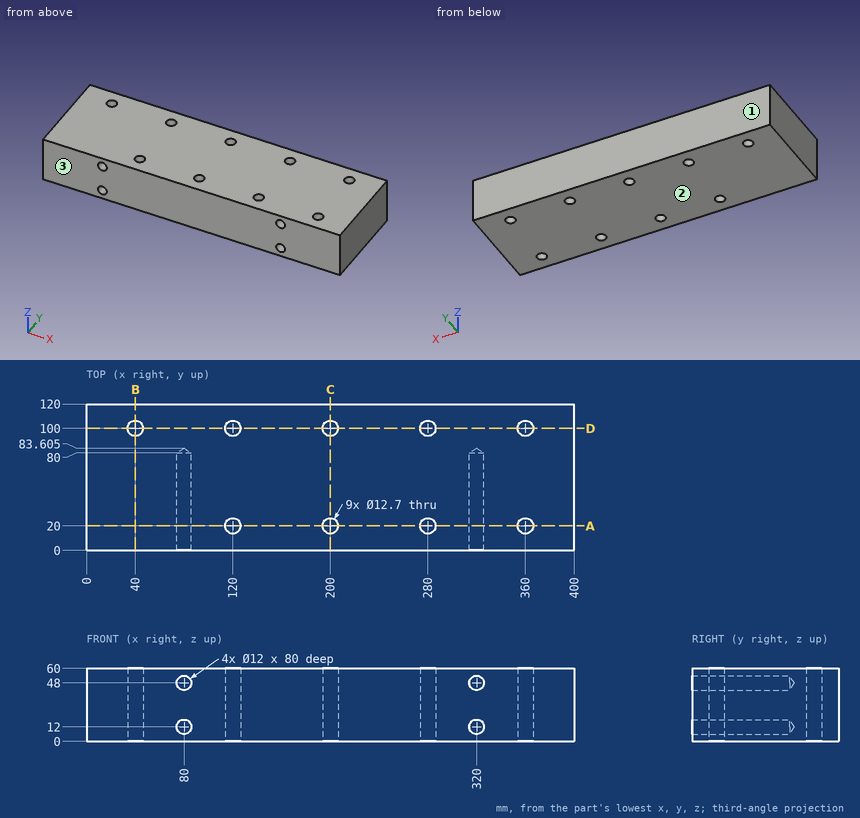
The drawing under review shows one solid part. Ordinate dimensions are in mm from its lowest x, y, z. Coordinates: 2 decimals unless noted, no trailing zeros. Order: outer loops, then holes, each group sorted by start corner. A loop starts at its lowest first (then second) coordinate and runs counter-clockwise, first axis right, second up. Notation, with made-up numbers: (8, 78) -> (48, 78) arc R20 cw to (48, 100) -> close; hole circle Ø8 at (-36, -31.75). An arc over 180 degrees is marked (long way). Answer in a Markdown table with one row per item. Add a question column.
Item 1: To check wall thickness, follow probe 1 along X at (y, z) = (56, 12); probe 2 along Z at (x, y) = (80, 62); probe 3 along Y at (x, z) = (360, 31). State the ranges of each line that lie inside material, in increasing order.
Item 2: Mouldability with a two-part tool opening along Y and no side actions: class the marked faces 1, 2 and 3 as +Y half, -Y half, draft (parallel to the pull), parting line (faces both ways), or undercut.
Item 3: We need section B-B on x = 40. Write out the cut boundary in (y, z).
Item 4: We need section D-D on y = 100. Write out the cut boundary in (x, z).
Item 5: We need section C-C on x = 200. Write out the cut boundary in (y, z), plus the area to 3 significant figures.
Item 6: We need section A-A on y = 20. Give the number of separate pieces and of enclosed holes in the cut face, plus the area to 3 significant figures.
Item 7: Clearance check with flat-ended pins moving along their axes: pin 1 (16.5 mm diameter, centred on x = 120, y = 20, fed in from -Z); pin 2 (7.5 mm diameter, centred on x = 200, y = 20, fed in from +Z); pin 3 (11 mm diameter, centred on x = 320, z = 48, fed in from -Y). State where each tip first meets the part, or that it passes through.
Final values:
| question | item | result |
|---|---|---|
| 1 | probe 1 | x = 0 to 74, 86 to 314, 326 to 400 |
| 1 | probe 2 | z = 0 to 6, 18 to 42, 54 to 60 |
| 1 | probe 3 | y = 0 to 13.65, 26.35 to 93.65, 106.35 to 120 |
| 2 | face 1 | +Y half |
| 2 | face 2 | draft |
| 2 | face 3 | -Y half |
| 3 | outline | (0, 0) -> (93.65, 0) -> (93.65, 60) -> (0, 60) -> close; (106.35, 0) -> (120, 0) -> (120, 60) -> (106.35, 60) -> close |
| 4 | outline | (0, 0) -> (33.65, 0) -> (33.65, 60) -> (0, 60) -> close; (46.35, 0) -> (113.65, 0) -> (113.65, 60) -> (46.35, 60) -> close; (126.35, 0) -> (193.65, 0) -> (193.65, 60) -> (126.35, 60) -> close; (206.35, 0) -> (273.65, 0) -> (273.65, 60) -> (206.35, 60) -> close; (286.35, 0) -> (353.65, 0) -> (353.65, 60) -> (286.35, 60) -> close; (366.35, 0) -> (400, 0) -> (400, 60) -> (366.35, 60) -> close |
| 5 | outline | (0, 0) -> (13.65, 0) -> (13.65, 60) -> (0, 60) -> close; (26.35, 0) -> (93.65, 0) -> (93.65, 60) -> (26.35, 60) -> close; (106.35, 0) -> (120, 0) -> (120, 60) -> (106.35, 60) -> close |
| 5 | area | 5,680 mm2 |
| 6 | separate pieces | 5 |
| 6 | enclosed holes | 4 |
| 6 | area | 20,500 mm2 |
| 7 | pin 1 | stops at z = 0 |
| 7 | pin 2 | passes through |
| 7 | pin 3 | stops at y = 80.3 |
